Part print with two shaded views. Sizes in mm from the minimum x, y, z corner. Give positions to 0.01 mm unless a question says otherwise; leave off trailing zeros. Order: outer loops, then holes, each group sorted by start corner. A loop starts at its lowest first (then second) coordinate and runs counter-clockwise, first axis right, second up. Notation, with made-up numbers: (-34.5, 4) -> (-12.5, 4) arc R18 cw to (-12.5, 17) -> close; hole circle Ø3 at (1, 23.5). An arc over 180 degrees is marked (long way). Write item = value, one per line. Start each with the question number.
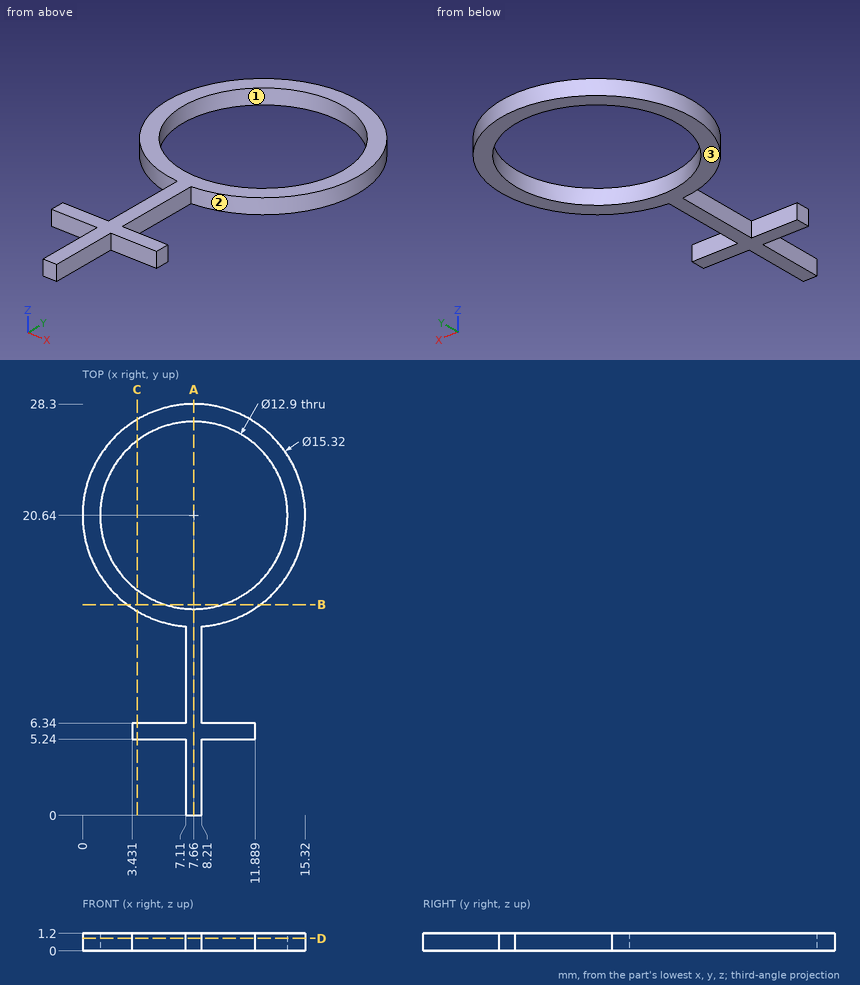
(1) Mould opens along X. For the marked faces 1, 2 and 3 say: released by +X, released by -X, zero draft, split by the parting line, or undercut.
(2) Cut at C-C, the plane x = 3.75. Give the cut face in (y, z).
(3) Flat gauge pins, fed straight in: P1, Ø0.6, axis at y = 10.5, z = 1, coming from the -X side; P2, Ø1.5, axis at x = 11.5, y = 19.5, coming from the -Z side; P3, Ø0.5, axis at y = 5.5, z = 0.5, coming from the -X side. Where does each tip first touch, or does it go through?
(4) Cut at D-D, the plane z = 0.85. Give the cut face in (x, y).
(5) Cut at B-B, the plane y = 14.5. Give the cut face in (x, z) (1 decimal).
(6) Wall check: line 1 (Y direction, x = 7.66, z = 0.85); line 2 (Y direction, x = 9, z = 1.1); line 3 (Y direction, x = 3.75, z = 0.7). Give the ranges that are in metal, low to high. Write a range as [from, to].
(7) Cut at A-A, the plane x = 7.66. Give the cut face in (y, z), plus the area to 3 significant figures.
Results:
q1.face_1 = undercut
q1.face_2 = split by the parting line
q1.face_3 = zero draft
q2.outline = (5.24, 0) -> (6.34, 0) -> (6.34, 1.2) -> (5.24, 1.2) -> close; (14.05, 0) -> (15.51, 0) -> (15.51, 1.2) -> (14.05, 1.2) -> close; (25.77, 0) -> (27.23, 0) -> (27.23, 1.2) -> (25.77, 1.2) -> close
q3.P1 = 7.11
q3.P2 = through
q3.P3 = 3.43
q4.outline = (3.43, 5.24) -> (7.11, 5.24) -> (7.11, 0) -> (8.21, 0) -> (8.21, 5.24) -> (11.89, 5.24) -> (11.89, 6.34) -> (8.21, 6.34) -> (8.21, 13) arc R7.66 ccw (long way) to (7.11, 13) -> (7.11, 6.34) -> (3.43, 6.34) -> close; hole circle Ø12.9 at (7.66, 20.64)
q5.outline = (3.1, 0) -> (5.7, 0) -> (5.7, 1.2) -> (3.1, 1.2) -> close; (9.6, 0) -> (12.2, 0) -> (12.2, 1.2) -> (9.6, 1.2) -> close
q6.line_1 = [0, 14.19], [27.09, 28.3]
q6.line_2 = [5.24, 6.34], [13.1, 14.33], [26.95, 28.18]
q6.line_3 = [5.24, 6.34], [14.05, 15.51], [25.77, 27.23]
q7.outline = (0, 0) -> (14.19, 0) -> (14.19, 1.2) -> (0, 1.2) -> close; (27.09, 0) -> (28.3, 0) -> (28.3, 1.2) -> (27.09, 1.2) -> close
q7.area = 18.5 mm2
